Input: part model. Units: mm. Frame: model coordinates. A direction names the side the tool comes from. Round coordinates to 2 decimals unless told otherwise and drop trailing zeros. Loops run counter-clockwise (first coordinate to the right, second up) from the corner with the lowest first, then second, coordinate; pieces in that order, holes last. Notation, with made-up numbers: M -21.75,-30.75 L 8.25,-30.75 A27 cw 8.25,-7.75 Z; hole C 81.25,-29 d7. An arc over 180 degrees is marked long. Return JSON: item names as keys, results as strings. Group by question number.
1) Material intervals for line 1 (X direction, y = 19.5, z = -1.8); line 2 (X direction, y = 19.5, z = -0.9); line 3 (Y direction, x = -36, z = -0.75), sorted ascending. Write a range as from..to.
2) Mould query, pull axis X, two halves, no side actions, for faces 3 (the face through (45.463, 18.839, -1.754)), 4 (the face through (-50.5, 1, -1)), 5 (the face through (-1, 1, -2)). Classes: +X half, -X half, draft (parallel to the pull), parting line (faces both ways), or undercut.
3) Section A-A (y = -19.5). Output: boundary loops of the cut face in (x, z), plus the area to 3 significant figures.
4) Section B-B (x = 46.5). Output: boundary loops of the cut face in (y, z).
5) Access query for faces 1 (the face through (27.157, -30.888, -1.014)), 2 (the face through (46, 18, -1.5)). Directions: +Z, -Z, +X, -X, +Y, -Y. A direction counts if a zero-diameter tool reaches every point of the face in a straight line with its end or side. Return the directions, or none.
6) Contact query for a flat-ended pin moving along its axis: P1, Ø3, axis at x = -46, y = -20, coming from the +Z side. Output: stop coordinate, or through.
7) Section C-C (z = -0.7). Count the separate pieces of the cut face and the enclosed holes in it, plus the area to 3 significant figures.
Autodesk Inventor part; units mm, degrees
ref_plane "YZ Plane" through (0, 0, 0) normal (1, 0, 0) x (0, 1, 0)
ref_plane "XZ Plane" through (0, 0, 0) normal (0, 1, 0) x (-1, 0, 0)
ref_plane "XY Plane" through (0, 0, 0) normal (0, 0, 1) x (1, 0, 0)
sketch "Esboço1" plane through (0, 0, 0) normal (0, 0, 1) x (1, 0, 0)
  line L0 (-50.5, -39) -> (50.5, -39)
  line L1 (50.5, -39) -> (50.5, 39)
  line L2 (50.5, 39) -> (-50.5, 39)
  line L3 (-50.5, 39) -> (-50.5, -39)
  point P0 (0, 0)
  dimension "d2" = 101
  dimension "d3" = 78
  dimension "d4" = 101
  dimension "d5" = 50.5
  dimension "d6" = 39
extrude "Extrusão1" add sketch "Esboço1" against normal blind 2
sketch "Esboço2" plane through (0, 0, 0) normal (0, 0, 1) x (1, 0, 0)
  line L0 (-50.5, -39) -> (-50.5, 39)
  line L1 (-42.5, -39) -> (-42.5, 39) construction
  line L2 (42.5, -39) -> (42.5, 39) construction
  line L3 (-46.5, 39) -> (-46.5, -39) construction
  line L4 (-50.5, 39) -> (50.5, 39)
  line L5 (46.5, 39) -> (46.5, -39) construction
  line L6 (50.5, 39) -> (50.5, -39)
  line L7 (-50.5, -19.5) -> (50.5, -19.5) construction
  line L8 (-50.5, 19.5) -> (50.5, 19.5) construction
  point P0 (0, 0)
  point P1 (-46.5, 19.5)
  point P2 (-46.5, -19.5)
  point P3 (46.5, -19.5)
  point P4 (46.5, 19.5)
hole "Furo1" at (-46.5, 19.5, 0) at (-46.5, -19.5, 0) at (46.5, -19.5, 0) at (46.5, 19.5, 0) direction (0, 0, -1) diameter 2.459 end through all counterbore diameter 6.5 counterbore depth 1.5
sketch "Esboço3" plane through (0, 0, -2) normal (0, 0, -1) x (-1, 0, 0)
  line L0 (39.7375, -31.6586) -> (-39.7375, -31.6586)
  line L1 (-29.1874, -30.9886) -> (-27.9874, -30.9886)
  line L2 (-27.9874, -30.9886) -> (-27.9374, -31.5336)
  line L3 (-29.1874, -30.9886) -> (-29.2374, -31.5336)
  line L4 (-22.5874, -30.9886) -> (-21.3874, -30.9886)
  line L5 (-22.5874, -30.9886) -> (-22.6374, -31.5336)
  line L6 (-21.3874, -30.9886) -> (-21.3374, -31.5336)
  line L7 (-21.3874, -30.9886) -> (-21.3874, -30.9886)
  line L8 (-15.9874, -30.9886) -> (-14.7874, -30.9886)
  line L9 (-15.9874, -30.9886) -> (-16.0374, -31.5336)
  line L10 (-14.7874, -30.9886) -> (-14.7374, -31.5336)
  line L11 (-9.3874, -30.9886) -> (-8.1874, -30.9886)
  line L12 (-8.1874, -30.9886) -> (-8.1374, -31.5336)
  line L13 (-9.3874, -30.9886) -> (-9.4374, -31.5336)
  line L14 (-2.7874, -30.9886) -> (-1.5874, -30.9886)
  line L15 (-2.7874, -30.9886) -> (-2.8374, -31.5336)
  line L16 (-1.5874, -30.9886) -> (-1.5374, -31.5336)
  line L17 (3.8127, -30.9886) -> (5.0127, -30.9886)
  line L18 (5.0127, -30.9886) -> (5.0627, -31.5336)
  line L19 (3.8127, -30.9886) -> (3.7627, -31.5336)
  line L20 (10.4126, -30.9886) -> (11.6126, -30.9886)
  line L21 (10.4126, -30.9886) -> (10.4126, -30.9886)
  line L22 (10.4126, -30.9886) -> (10.3626, -31.5336)
  line L23 (11.6126, -30.9886) -> (11.6626, -31.5336)
  line L24 (17.0126, -30.9886) -> (18.2126, -30.9886)
  line L25 (17.0126, -30.9886) -> (16.9626, -31.5336)
  line L26 (18.2126, -30.9886) -> (18.2626, -31.5336)
  line L27 (35.0474, -31.0186) -> (35.9774, -31.0186)
  line L28 (36.3874, -31.6586) -> (36.3874, -31.0186)
  line L29 (34.6374, -31.6586) -> (34.6374, -31.0186)
  line L30 (35.0474, -31.0186) -> (34.6374, -31.0186)
  line L31 (36.3874, -31.0186) -> (35.9774, -31.0186)
  line L32 (-28.5874, -31.3386) -> (36.3874, -31.3386) construction
  circle A0 centre (35.5124, -31.3386) radius 1.5
  circle A1 centre (-28.5874, -31.3386) radius 1.5
  circle A2 centre (17.6126, -31.3386) radius 1.5
  circle A3 centre (11.0126, -31.3386) radius 1.5
  circle A4 centre (4.4127, -31.3386) radius 1.5
  circle A5 centre (-2.1874, -31.3386) radius 1.5
  circle A6 centre (-8.7874, -31.3386) radius 1.5
  circle A7 centre (-15.3874, -31.3386) radius 1.5
  circle A8 centre (-21.9874, -31.3386) radius 1.5
  point P0 (0, 0)
  dimension "d23" = 3
  dimension "d24" = 3
  dimension "d25" = 3
  dimension "d26" = 3
  dimension "d27" = 3
  dimension "d28" = 3
  dimension "d29" = 3
  dimension "d30" = 3
  dimension "d31" = 3
  dimension "d32" = 0.32
  dimension "d33" = 0.875
  dimension "d34" = 18.7748
  dimension "d35" = 25.3748
  dimension "d36" = 31.9748
  dimension "d37" = 38.5748
  dimension "d38" = 45.1748
  dimension "d39" = 51.7748
  dimension "d40" = 58.3748
  dimension "d41" = 64.9748
extrude "Extrusão2" cut sketch "Esboço3" against normal blind 10
properties part number "Ra-Manager_Painel-Placas_Relays" material "Aço, carbono"
Returned:
{
 "1": {"line 1": "x = -50.5..-47.73, -45.27..45.27, 47.73..50.5", "line 2": "x = -50.5..-49.75, -43.25..43.25, 49.75..50.5", "line 3": "y = -39..-32.76, -29.92..39"},
 "2": {"face 3": "undercut", "face 4": "-X half", "face 5": "draft"},
 "3": {"outline": "M -50.5,-2 L -47.73,-2 L -47.73,-1.5 L -49.75,-1.5 L -49.75,0 L -50.5,0 Z; M -45.27,-2 L 45.27,-2 L 45.27,-1.5 L 43.25,-1.5 L 43.25,0 L -43.25,0 L -43.25,-1.5 L -45.27,-1.5 Z; M 47.73,-2 L 50.5,-2 L 50.5,0 L 49.75,0 L 49.75,-1.5 L 47.73,-1.5 Z", "area": "180 mm^2"},
 "4": {"outline": "M -39,-2 L -20.73,-2 L -20.73,-1.5 L -22.75,-1.5 L -22.75,0 L -39,0 Z; M -18.27,-2 L 18.27,-2 L 18.27,-1.5 L 16.25,-1.5 L 16.25,0 L -16.25,0 L -16.25,-1.5 L -18.27,-1.5 Z; M 20.73,-2 L 39,-2 L 39,0 L 22.75,0 L 22.75,-1.5 L 20.73,-1.5 Z"},
 "5": {"face 1": "+Z, -Z", "face 2": "+Z"},
 "6": {"P1": "stops at z = -1.5"},
 "7": {"separate pieces": "1", "enclosed holes": "13", "area": "7,680 mm^2"}
}
